from build123d import *

# Parameters (mm, degrees)
SKETCH1_W                                           = 250
SKETCH1_H                                           = 149.999999994
BOSS_EXTRUDE1_DEPTH                                 = 12.7
CBORE_FOR_8_BINDING_HEAD_MACHINE_SCREW1_D           = 4.4958
CBORE_FOR_8_BINDING_HEAD_MACHINE_SCREW1_CBORE_D     = 9.525
CBORE_FOR_8_BINDING_HEAD_MACHINE_SCREW1_CBORE_DEPTH = 4.445
F_1_4_20_TAPPED_HOLE1_D                             = 5.1054
CUT_EXTRUDE1_DEPTH                                  = 8
FILLET1_R                                           = 4.999999906
FILLET1_OF_MIRROR1_R                                = 4.999999906
CUT_EXTRUDE3_DEPTH                                  = 8
FILLET3_R                                           = 4.999999906
CUT_EXTRUDE4_DEPTH                                  = 147.325971719
CUT_EXTRUDE5_DEPTH                                  = 4.445


with BuildPart() as part:
    # Sketch1 → Boss-Extrude1 (new body)
    with BuildSketch(Plane(origin=(0, 0, 0), x_dir=(1, 0, 0), z_dir=(0, 1, 0))):
        Rectangle(SKETCH1_W, SKETCH1_H)
    extrude(amount=BOSS_EXTRUDE1_DEPTH)

    # CBORE for #8 Binding Head Machine Screw1 (through all)
    with Locations(Plane.XZ):
        with Locations((-30, 43.249999997), (30, 43.249999997), (0, 0.069999997), (-105, -26.750000003), (-90, -26.750000003), (-90, -6.750000003), (-105, -6.750000003), (-10, -66.929999703), (10, -66.929999703)):
            cbore_for_8_binding_head_machine_screw1 = CounterBoreHole(CBORE_FOR_8_BINDING_HEAD_MACHINE_SCREW1_D / 2, CBORE_FOR_8_BINDING_HEAD_MACHINE_SCREW1_CBORE_D / 2, CBORE_FOR_8_BINDING_HEAD_MACHINE_SCREW1_CBORE_DEPTH)

    # 1/4-20 Tapped Hole1 (through all)
    with Locations(Plane.XZ):
        with Locations((100, -49.999999997), (-100, -49.999999997), (-100, 49.999999997), (100, 49.999999997)):
            Hole(F_1_4_20_TAPPED_HOLE1_D / 2)

    # Sketch10 → Cut-Extrude1 (cut)
    with BuildSketch(Plane(origin=(0, 12.7, 0), x_dir=(1, 0, 0), z_dir=(0, 1, 0))):
        Polygon((-80, 64.999999997), (-80, -1.200000003), (-115, -1.200000003), (-115, -43.249999997), (-85, -43.249999997), (-85, -64.999999997), (-65.655144454, -64.999999997), (-48.8, -24.999999997), (-36.1, -24.999999997), (-15.78, 64.999999997), align=None)
    cut_extrude1 = extrude(amount=-CUT_EXTRUDE1_DEPTH, mode=Mode.SUBTRACT)

    # Fillet1
    fillet1_edges = [part.edges().sort_by_distance(p)[0] for p in [
        (-15.78, 8.7, -64.999999997),
        (-36.1, 8.7, 24.999999997),
        (-48.8, 8.7, 24.999999997),
        (-65.655144454, 8.7, 64.999999997),
        (-85, 8.7, 64.999999997),
        (-85, 8.7, 43.249999997),
        (-115, 8.7, 43.249999997),
        (-115, 8.7, 1.200000003),
        (-80, 8.7, 1.200000003),
        (-80, 8.7, -64.999999997),
    ]]
    fillet(fillet1_edges, radius=FILLET1_R)

    # Mirror1: Cut-Extrude1 across plane
    add(cut_extrude1.mirror(Plane(origin=(0, 0, 0), x_dir=(0, 0, 1), z_dir=(1, 0, 0))), mode=Mode.SUBTRACT)

    # Fillet1 of Mirror1
    fillet1_of_mirror1_edges = [part.edges().sort_by_distance(p)[0] for p in [
        (15.78, 8.7, -64.999999997),
        (36.1, 8.7, 24.999999997),
        (48.8, 8.7, 24.999999997),
        (65.655144454, 8.7, 64.999999997),
        (85, 8.7, 64.999999997),
        (85, 8.7, 43.249999997),
        (115, 8.7, 43.249999997),
        (115, 8.7, 1.200000003),
        (80, 8.7, 1.200000003),
        (80, 8.7, -64.999999997),
    ]]
    fillet(fillet1_of_mirror1_edges, radius=FILLET1_OF_MIRROR1_R)

    # Sketch14 → Cut-Extrude3 (cut)
    with BuildSketch(Plane(origin=(0, 12.7, 0), x_dir=(1, 0, 0), z_dir=(0, 1, 0))):
        Polygon((-54.905605596, -64.999999997), (54.905605596, -64.999999997), (48.584926426, -49.999999997), (-48.584926426, -49.999999997), align=None)
    extrude(amount=-CUT_EXTRUDE3_DEPTH, mode=Mode.SUBTRACT)

    # Fillet3
    fillet3_edges = [part.edges().sort_by_distance(p)[0] for p in [
        (-54.905605596, 8.7, 64.999999997),
        (-48.584926426, 8.7, 49.999999997),
        (48.584926426, 8.7, 49.999999997),
        (54.905605596, 8.7, 64.999999997),
    ]]
    fillet(fillet3_edges, radius=FILLET3_R)

    # Sketch15 → Cut-Extrude4 (cut, through all)
    with BuildSketch(Plane(origin=(0, 12.7, 0), x_dir=(1, 0, 0), z_dir=(0, 1, 0))):
        with BuildLine():
            Line((-36, -41.002099997), (-24, -41.002099997))
            ThreePointArc((-24, -41.002099997), (-21.7521, -43.249999997), (-24, -45.497899997))
            Line((-24, -45.497899997), (-36, -45.497899997))
            ThreePointArc((-36, -45.497899997), (-38.2479, -43.249999997), (-36, -41.002099997))
        make_face()
        with BuildLine():
            Line((24, -41.002099997), (36, -41.002099997))
            ThreePointArc((36, -41.002099997), (38.2479, -43.249999997), (36, -45.497899997))
            Line((36, -45.497899997), (24, -45.497899997))
            ThreePointArc((24, -45.497899997), (21.7521, -43.249999997), (24, -41.002099997))
        make_face()
        with BuildLine():
            Line((2.2479, 5.930000003), (2.2479, -6.069999997))
            ThreePointArc((2.2479, -6.069999997), (0, -8.317899997), (-2.2479, -6.069999997))
            Line((-2.2479, -6.069999997), (-2.2479, 5.930000003))
            ThreePointArc((-2.2479, 5.930000003), (0, 8.177900003), (2.2479, 5.930000003))
        make_face()
    extrude(amount=-CUT_EXTRUDE4_DEPTH, mode=Mode.SUBTRACT)

    # Sketch16 → Cut-Extrude5 (cut)
    with BuildSketch(Plane.XZ):
        with BuildLine():
            Line((-4.7625, -6), (-4.7625, 6))
            ThreePointArc((-4.7625, 6), (0, 10.7625), (4.7625, 6))
            Line((4.7625, 6), (4.7625, -6))
            ThreePointArc((4.7625, -6), (0, -10.7625), (-4.7625, -6))
        make_face()
        with BuildLine():
            Line((36, 38.487499997), (24, 38.487499997))
            ThreePointArc((24, 38.487499997), (19.2375, 43.249999997), (24, 48.012499997))
            Line((24, 48.012499997), (36, 48.012499997))
            ThreePointArc((36, 48.012499997), (40.7625, 43.249999997), (36, 38.487499997))
        make_face()
        with BuildLine():
            Line((-24, 38.487499997), (-36, 38.487499997))
            ThreePointArc((-36, 38.487499997), (-40.7625, 43.249999997), (-36, 48.012499997))
            Line((-36, 48.012499997), (-24, 48.012499997))
            ThreePointArc((-24, 48.012499997), (-19.2375, 43.249999997), (-24, 38.487499997))
        make_face()
    extrude(amount=-CUT_EXTRUDE5_DEPTH, mode=Mode.SUBTRACT)

    # Mirror3: CBORE for #8 Binding Head Machine Screw1 across plane
    add(cbore_for_8_binding_head_machine_screw1.mirror(Plane(origin=(0, 0, 0), x_dir=(0, 0, 1), z_dir=(1, 0, 0))), mode=Mode.SUBTRACT)


solid = part.part
Read the model definition and answer for the solid it produces. Units are mm, in the model's axes. A direction names the side the tool comes from. Round coordinates to 2 decimals unless told otherwise and drop trailing zeros. Loops run counter-clockwise (first coordinate to the right, second up) from the corner with the lowest first, then second, coordinate; pieces in that order, holes last. Notation, with made-up numbers: (38, 72) - (43, 72) arc R11 cw to (43, 91) - close; hole circle Ø11 at (1.5, 46). An arc over 180 degrees is marked (long way). One line per question, with ' | ' between items. Start each with the question number.
Q1. Section A-A on x = -31.5 is taken. Give the vertices of the cut face in (y, z) (1 decimal), plus the area to 3 significant figures.
Q2. For a pull along X with two mould halves and no side action, classify faces 1 (the flat face through (-2, 6, 75)), 2 (the cylindrical face through (51.5, 8.64, 62.82)) as +X half, -X half, draft (parallel to the pull), parting line (faces both ways), or undercut.
Q3. Flat-ended cylindrical pins translate along their axes: pin 1 (10.5 mm diameter, centred on x = -92, z = -26.5, fed in from -Y); pin 2 (5 mm diameter, centred on x = 90, z = -26.75, fed in from -Y) (3 decimals); pin 3 (4.5 mm diameter, centred on x = -2.5, z = 59, fed in from +Y). Find the tip coordinate at first contact, or state that the pin passes through.
Q4. For faces 3 (the cylindrical face through (94.758, 2.191, -6.541)), 4 (the flat face through (-2.248, 9, 0)), 5 (the cylindrical face through (86.43, 8.64, 44.75)), 6 (the flat face through (-2, 6, -75)), determine the directions among +Z, -Z, +X, -X, +Y, -Y from which every point of the face is accessible in a straight line to the end or side of a thin tool.
Q5. Find the intervals of material crossed by L1, parallel to Z at x = 90, y = 10.25; L2, parallel to Z at x = -42, y = 11; L3, parallel to Z at x = -90, y = 1.6, in increasing order.
Q6. Section B-B on z = -50 is taken. Give the vertices of the cut face in (x, y).
Q7. Section C-C on y = 7 is taken. Count the separate pieces of the cut face and the enclosed holes in it, plus the area to 3 significant figures.
Established:
1) outline: (0, -75) - (12.7, -75) - (12.7, -65) - (4.7, -65) - (4.7, 4.6) - (12.7, 4.6) - (12.7, 41) - (4.4, 41) - (4.4, 38.5) - (0, 38.5) - close; (0, 48) - (4.4, 48) - (4.4, 45.5) - (12.7, 45.5) - (12.7, 50) - (4.7, 50) - (4.7, 65) - (12.7, 65) - (12.7, 75) - (0, 75) - close | area: 1,150 mm²
2) face 1: draft | face 2: undercut
3) pin 1: y = 0 | pin 2: y = 4.445 | pin 3: y = 4.7
4) face 3: -Y | face 4: +Y, -Y | face 5: +Y | face 6: -Z, +X, -X, +Y, -Y
5) L1: -75 to -29, -24.5 to -9, -4.5 to 1.2, 43.25 to 75 | L2: -75 to -65, 25 to 50, 65 to 75 | L3: -75 to -31.51, -21.99 to -11.51, -1.99 to 75
6) outline: (-125, 0) - (-102.55, 0) - (-102.55, 12.7) - (-125, 12.7) - close; (-97.45, 0) - (97.45, 0) - (97.45, 12.7) - (80, 12.7) - (80, 4.7) - (19.17, 4.7) - (19.17, 12.7) - (-19.17, 12.7) - (-19.17, 4.7) - (-80, 4.7) - (-80, 12.7) - (-97.45, 12.7) - close; (102.55, 0) - (125, 0) - (125, 12.7) - (102.55, 12.7) - close
7) separate pieces: 1 | enclosed holes: 20 | area: 20,900 mm²
